Autodesk Inventor part; units mm, degrees
ref_plane "YZ Plane" through (0, 0, 0) normal (1, 0, 0) x (0, 1, 0)
ref_plane "XZ Plane" through (0, 0, 0) normal (0, 1, 0) x (-1, 0, 0)
ref_plane "XY Plane" through (0, 0, 0) normal (0, 0, 1) x (1, 0, 0)
sketch "Sketch2" plane through (0, 0, 0) normal (0, 0, 1) x (1, 0, 0)
  line L0 (-12.7, -12.7) -> (12.7, -12.7)
  line L1 (12.7, -12.7) -> (12.7, 12.7)
  line L2 (12.7, 12.7) -> (-12.7, 12.7)
  line L3 (-12.7, 12.7) -> (-12.7, -12.7)
  line L4 (-12.7, -12.7) -> (12.7, 12.7) construction
  line L5 (12.7, -12.7) -> (-12.7, 12.7) construction
  line L6 (-9.525, -9.525) -> (9.525, -9.525)
  line L7 (9.525, -9.525) -> (9.525, 9.525)
  line L8 (9.525, 9.525) -> (-9.525, 9.525)
  line L9 (-9.525, 9.525) -> (-9.525, -9.525)
  line L10 (-9.525, -9.525) -> (9.525, 9.525) construction
  line L11 (9.525, -9.525) -> (-9.525, 9.525) construction
  point P0 (0, 0)
  dimension "d0" = 25.4
  dimension "d1" = 25.4
  dimension "d2" = 3.175
  dimension "d3" = 3.175
extrude "Extrusion1" add sketch "Sketch2" along normal mid plane 879.856
sketch "Sketch3" plane through (12.7, -12.7, 439.928) normal (1, 0, 0) x (0, 0, -1)
  line L0 (879.856, 25.4) -> (879.856, 0)
  line L1 (879.856, 25.4) -> (865.1913, 0)
  line L2 (879.856, 0) -> (0, 0)
  line L3 (865.1913, 0) -> (879.856, 0)
  line L4 (879.856, 25.4) -> (0, 25.4)
  line L5 (879.856, 0) -> (879.856, 25.4)
  point P0 (439.928, 12.7)
  dimension "d6" = 30
extrude "Extrusion2" cut sketch "Sketch3" against normal through all
sketch "Sketch4" plane through (12.7, -12.7, 439.928) normal (1, 0, 0) x (0, 0, -1)
  line L0 (0, 25.4) -> (0, 0)
  line L1 (0, 25.4) -> (36.2286, 4.4834)
  line L2 (36.2286, 4.4834) -> (43.9941, 0)
  line L3 (865.1913, 0) -> (0, 0)
  line L4 (0, 25.4) -> (0, 0)
  line L5 (0, 0) -> (43.9941, 0)
  point P0 (439.928, 12.7)
  dimension "d9" = 60
extrude "Extrusion3" cut sketch "Sketch4" against normal through all
properties part number "aluminumBallHandlerHypotenuse" material "Aluminum 6061-AHC"
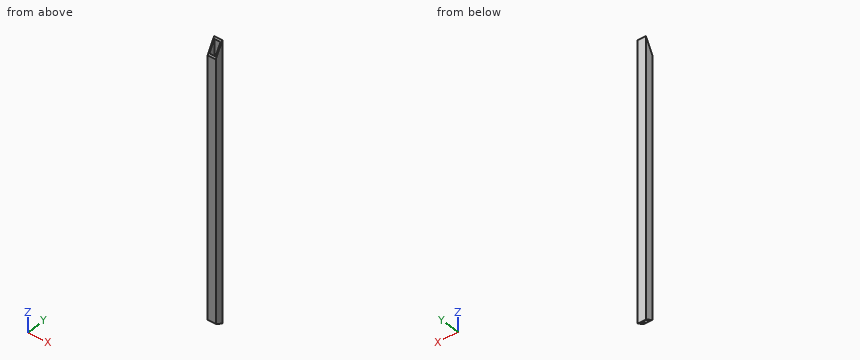
Could you check a few things on this model? Use its own coordinates, in mm. Round coordinates to 2 decimals unless told otherwise and drop trailing zeros. Write each loop counter-clockwise with the first axis right and the second up, starting at its lowest first coordinate (ties: lowest second). Pieces come first, ordered by that corner, then holes. Notation, with made-up numbers: M 13,-4.5 L 18,-4.5 A26 cw 18,26.5 Z; hole C 57,65.25 d10. An arc over 180 degrees is marked long. Write each question's results on one line, items separated by ' | '. Start each with the question number.
1. Imagine slicing it at A-A on x = -2. List the corners of the cut face in (y, z) for me (3 decimals), and give its area (3 significant figures).
2. Imagine slicing it at B-B on z = -381.5. List the corners of the cut face in (x, y) for me (3 decimals).
3. I'm going to push flat-ended pins straight in: pin 1 Ø10 at (x, y) = (9.5, 5.5) entering from -Z; pin 2 Ø5 at (x, y) = (10, -5) entering from +Z; pin 3 Ø4 at (x, y) = (-9.5, -5) entering from -Z. Where does each tip first touch, or does it pass through?
4. I need wall thicknesses on L1, parallel to Y at x = -4.75, z = -42 (3 decimals); L2, parallel to Z at x = -10, y = 9.5. Which ranges of each line are inside material? Lowest first, please. Write a range as from..to.
5. Imagine slicing it at C-C on y = 0.75. List the corners of the cut face in (x, z) for me (3 decimals).
Result sheet:
1) outline: M -12.7,-425.263 L -9.525,-427.096 L -9.525,401.433 L -12.7,395.934 Z; M 9.525,-438.095 L 12.7,-439.928 L 12.7,439.928 L 9.525,434.429 Z | area: 5,400 mm^2
2) outline: M -12.7,-12.7 L 12.7,-12.7 L 12.7,12.7 L -12.7,12.7 Z; hole M -9.525,-9.525 L 9.525,-9.525 L 9.525,9.525 L -9.525,9.525 Z
3) pin 1: stops at z = -438.66 | pin 2: stops at z = 413.6 | pin 3: stops at z = -430.86
4) L1: y = -12.7..-9.525, 9.525..12.7 | L2: z = -438.08..434.39
5) outline: M -12.7,-433.029 L -9.525,-433.029 L -9.525,419.23 L -12.7,419.23 Z; M 9.525,-433.029 L 12.7,-433.029 L 12.7,419.23 L 9.525,419.23 Z
